The figure shows three views and two pictorial views of one solid part (mm, origin at its lowest corner). Answer the questions. Give positions to 0.01 mm unless a question says otherwise; leave off trailing zeros. Order: outer loops, then holes, each group sorted by start corner. A loop starts at its lowest first (then second) coordinate and runs counter-clockwise, first axis right, second up. Notation, with made-up numbers: (-2.5, 50) - (23.5, 50) arc R31 cw to (23.5, 87) - close; hole circle Ø2 at (78, 75.5). An arc over 180 degrees is marked (long way). Answer as a JSON object with one key per item and string values. Group by question number.
Q1. A cutting plane is placed at C-C, the plane z = 32. Give the vertices of the cut face in (x, y).
Q2. Consider line 1 (Z direction, x = 14, y = 10.5); line 2 (X direction, y = 9.25, z = 66); line 3 (Y direction, x = 11.75, z = 4.5). Determine where each line is inside the solid, lowest interval first.
Q3. The mould has two halves that part along Z. Classify the marked faces 1, 2, 3 and 4: released by +Z, released by -Z, zero draft, split by the parting line, or undercut.
Q4. A cutting plane is placed at B-B, the plane x = 1.5. Give the vertices of the cut face in (y, z), and give its area (3 significant figures).
Q5. Given pin 1 (3 mm diameter, centred on x = 10, z = 21, fed in from +Y); pin 2 (8 mm diameter, centred on y = 8, z = 42.5, fed in from +X); pin 3 (5 mm diameter, centred on x = 13.5, z = 33.5, fed in from -Y), each flat-ended and moving along its own axis, determine where each tip first touches the part or whether it passes through.
Q6. A cutting plane is placed at A-A, the plane y = 13. Give the vertices of the cut face in (x, z).
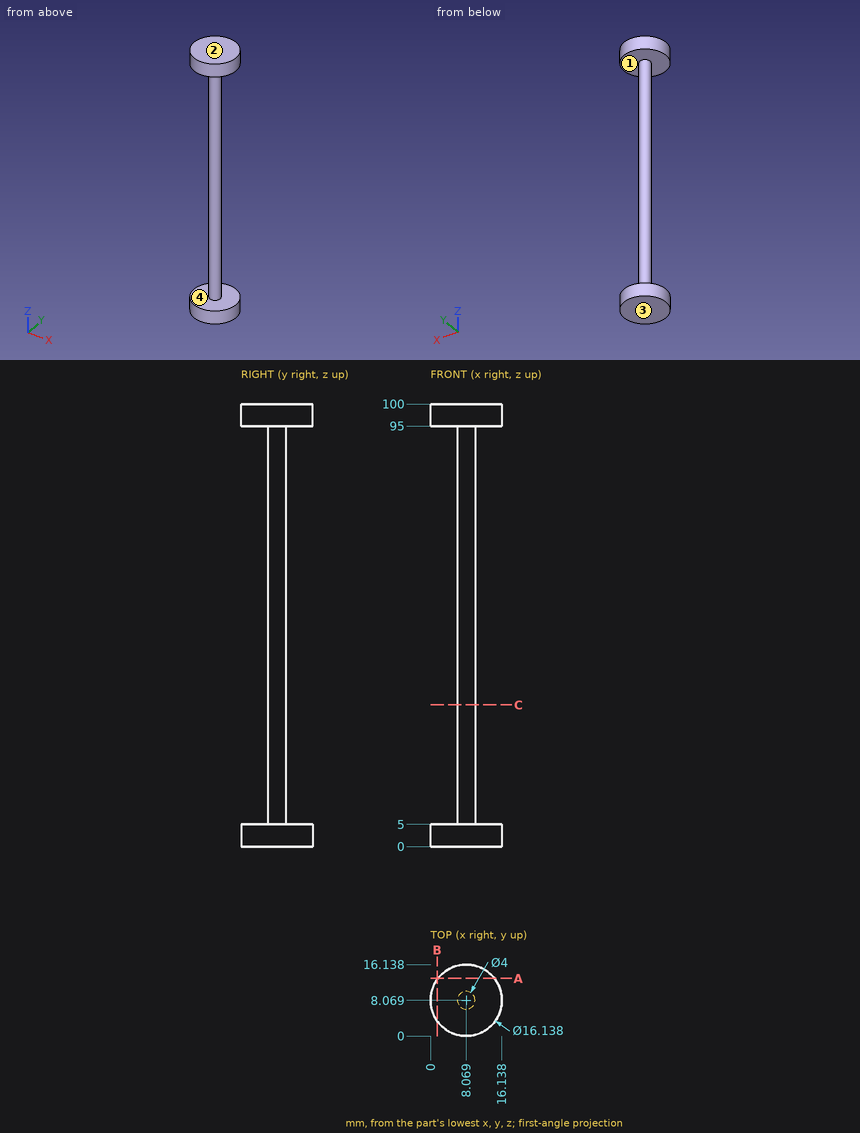
Reply:
{
 "1": {"outline": "circle Ø4 at (8.07, 8.07)"},
 "2": {"line 1": "z = 0 to 5, 95 to 100", "line 2": "x = 6.45 to 9.68", "line 3": "y = 0.89 to 15.25"},
 "3": {"face 1": "undercut", "face 2": "released by +Z", "face 3": "released by -Z", "face 4": "undercut"},
 "4": {"outline": "(3.38, 0) - (12.75, 0) - (12.75, 5) - (3.38, 5) - close; (3.38, 95) - (12.75, 95) - (12.75, 100) - (3.38, 100) - close", "area": "93.7 mm^2"},
 "5": {"pin 1": "stops at y = 10.02", "pin 2": "stops at x = 10.07", "pin 3": "passes through"},
 "6": {"outline": "(1.68, 0) - (14.46, 0) - (14.46, 5) - (1.68, 5) - close; (1.68, 95) - (14.46, 95) - (14.46, 100) - (1.68, 100) - close"}
}
